from build123d import *

# Parameters (mm, degrees)
SKETCH_1_R                  = 11.1
SKETCH_1_R_2                = 2
SKETCH_1_R_3                = 1.7
F_08_TILT_IDLER_CHEEK_DEPTH = 6


with BuildPart() as part:
    # Эскиз1 → 08_Tilt_idler_cheek (new body)
    with BuildSketch(Plane.XY):
        Polygon((-38, 0), (38, 0), (38, 62), (22, 88), (-22, 88), (-38, 62), align=None)
        with Locations((0, 57)):
            Circle(SKETCH_1_R, mode=Mode.SUBTRACT)
        with Locations((-24, 10)):
            Circle(SKETCH_1_R_2, mode=Mode.SUBTRACT)
        with Locations((24, 10)):
            Circle(SKETCH_1_R_3, mode=Mode.SUBTRACT)
    extrude(amount=F_08_TILT_IDLER_CHEEK_DEPTH)


solid = part.part
Build history of the part. All positions in model axes, mm. Round coordinates to 2 decimals unless told otherwise and drop trailing zeros. Order: outer loops, then holes, each group sorted by start corner. A loop starts at its lowest first (then second) coordinate and runs counter-clockwise, first axis right, second up. Notation, with made-up numbers: M -10,-17 L 36,-17 A17 ccw 36,8 Z; hole C 1.5,63 d7. An arc over 180 degrees is marked long. Use CSV: the item, a comma, the result in double quotes. Start each with the question number.
(1) Cut at A-A on y = 10. List the corners of the cut face in (x, z).
(2) Drill centre lines: probe 1 along Y at (x, z) = (0, 3.4); probe 2 along Y at (x, z) = (24, 2.5); probe 3 along X at (y, z) = (55.5, 0.85). Where is each one in solid material? Low to high.
(3) Mould opens along Y. For faces 1 (the face through (-2.406, 46.164, 2.958)), 2 (the face through (25.57, 9.35, 2.96)), 3 (the face through (-1, 45, 6)), 4 (the face through (0, 88, 3)) say: +Y half, -Y half, draft (parallel to the pull), parting line (faces both ways), or undercut.
(4) Cut at B-B on x = 0. List the corners of the cut face in (y, z).
(5) Cut at D-D on z = 4.6. List the corners of the cut face in (x, y), then the cut area to 3 significant figures.
(6) Flat gauge pin, fed straight in: P1, Ø12, axis at x = -10, y = 47, coming from the -Z side. Where does the tip first touch, or does it go through?
(7) Cut at C-C on y = 57. List the corners of the cut face in (x, z).
Findings:
1,outline,"M -38,0 L -26,0 L -26,6 L -38,6 Z; M -22,0 L 22.3,0 L 22.3,6 L -22,6 Z; M 25.7,0 L 38,0 L 38,6 L 25.7,6 Z"
2,probe 1,"y = 0 to 45.9, 68.1 to 88"
2,probe 2,"y = 0 to 8.3, 11.7 to 84.75"
2,probe 3,"x = -38 to -11, 11 to 38"
3,face 1,"undercut"
3,face 2,"undercut"
3,face 3,"draft"
3,face 4,"+Y half"
4,outline,"M 0,0 L 45.9,0 L 45.9,6 L 0,6 Z; M 68.1,0 L 88,0 L 88,6 L 68.1,6 Z"
5,outline,"M -38,0 L 38,0 L 38,62 L 22,88 L -22,88 L -38,62 Z; hole C -24,10 d4; hole C 0,57 d22.2; hole C 24,10 d3.4"
5,area,"5,860 mm^2"
6,P1,"stops at z = 0"
7,outline,"M -38,0 L -11.1,0 L -11.1,6 L -38,6 Z; M 11.1,0 L 38,0 L 38,6 L 11.1,6 Z"
